Source: CAD feature listing. Evaluate the final solid. Frame: model axes, mm. A direction names the side the tool comes from. Round coordinates to 2 decimals unless told otherwise and drop trailing zeros. Loops run counter-clockwise (first coordinate to the right, second up) from the corner with the lowest first, then second, coordinate; pieces in that order, holes last. Notation, with made-up numbers: (11, -34.5) - (41, -34.5) arc R16 ccw to (41, -28.5) - close; hole circle Ø7 at (-32, -11.75). An arc over 180 degrees is marked (long way). One line per question, with ' | ' between items.
Autodesk Inventor part; units mm, degrees
ref_plane "YZ Plane" through (0, 0, 0) normal (1, 0, 0) x (0, 1, 0)
ref_plane "XZ Plane" through (0, 0, 0) normal (0, 1, 0) x (-1, 0, 0)
ref_plane "XY Plane" through (0, 0, 0) normal (0, 0, 1) x (1, 0, 0)
sketch "Sketch1" plane through (0, 0, 0) normal (0, 1, 0) x (-1, 0, 0)
  line L0 (-12.7, 12.7) -> (12.7, 12.7)
  line L1 (12.7, 12.7) -> (12.7, -12.7)
  line L2 (12.7, -12.7) -> (-12.7, -12.7)
  line L3 (-12.7, -12.7) -> (-12.7, 12.7)
  line L4 (-12.7, 12.7) -> (12.7, -12.7) construction
  line L5 (12.7, 12.7) -> (-12.7, -12.7) construction
  line L6 (11.1125, -11.1125) -> (11.1125, 11.1125)
  line L7 (11.1125, 11.1125) -> (-11.1125, 11.1125)
  line L8 (-11.1125, 11.1125) -> (-11.1125, -11.1125)
  line L9 (-11.1125, -11.1125) -> (11.1125, -11.1125)
  point P0 (0, 0)
  dimension "d0" = 25.4
  dimension "d1" = 1.5875
extrude "Extrusion1" add sketch "Sketch1" along normal mid plane 1016
sketch "Sketch2" plane through (12.7, -508, -12.7) normal (1, 0, 0) x (0, 0, -1)
  circle A0 centre (-12.7, 12.7) radius 3.175
  line L0 (-12.7, 12.7) -> (-12.7, 0) construction
  line L1 (-23.8125, 0) -> (-1.5875, 0) construction
  point P0 (-12.7, 508)
  dimension "d4" = 6.35
  dimension "d5" = 12.7
extrude "Extrusion2" cut sketch "Sketch2" against normal through all
properties part number "climb bar"
1. Contact query for a flat-ended pin moving along its axis: P1, Ø8, axis at x = -1, z = -9.5, coming from the +Y side. Output: stop coordinate, or through.
Worked out:
P1: stops at y = 508
2. Access query for faces 4 (the flat face through (11.3, -508, 0.1)), 5 (the flat face through (0, -7, -11.112)). Directions: +Z, -Z, +X, -X, +Y, -Y. A direction counts if a zero-diameter tool reaches every point of the face in a straight line with its end or side. Return the directions, or none.
Worked out:
face 4: +Z, -Z, +X, -X, -Y | face 5: +Y, -Y
3. Material intervals for probe 1 along Y at (x, z) = (12.15, 0) (3 decimals); probe 2 along X at (y, z) = (-394, -2.5), sorted ascending.
Worked out:
probe 1: y = -508 to -498.475, -492.125 to 508 | probe 2: x = -12.7 to -11.11, 11.11 to 12.7
4. Section query A-A, the plane z = -7. Return loops of the section in (x, y).
Worked out:
outline: (-12.7, -508) - (-11.11, -508) - (-11.11, 508) - (-12.7, 508) - close; (11.11, -508) - (12.7, -508) - (12.7, 508) - (11.11, 508) - close
5. Section query B-B, the plane x = -5. Return loops of the section in (y, z).
Worked out:
outline: (-508, -12.7) - (508, -12.7) - (508, -11.11) - (-508, -11.11) - close; (-508, 11.11) - (508, 11.11) - (508, 12.7) - (-508, 12.7) - close
6. Section query C-C, the plane y = 410. Return loops of the section in (x, z), plus the area to 3 significant figures.
Worked out:
outline: (-12.7, -12.7) - (12.7, -12.7) - (12.7, 12.7) - (-12.7, 12.7) - close; hole (-11.11, -11.11) - (11.11, -11.11) - (11.11, 11.11) - (-11.11, 11.11) - close | area: 151 mm2
7. Mould query, pull axis X, two halves, no side actions, for faces 1 (the flat face through (-12.7, -7, 0)), 2 (the flat face through (11.112, -7, 0)), 3 (the flat face through (11.3, 508, 0.1)). Classes: released by +X, released by -X, zero draft, split by the parting line, or undercut.
Worked out:
face 1: released by -X | face 2: undercut | face 3: zero draft
